from build123d import *

# Parameters (mm, degrees)
SKETCH1_R           = 1
BOSS_EXTRUDE1_DEPTH = 7
SKETCH1_3_R         = 1
BOSS_EXTRUDE2_DEPTH = 2
CUT_EXTRUDE1_DEPTH  = 9
CUT_EXTRUDE2_DEPTH  = 9
FILLET1_R           = 1
FILLET2_R           = 0.3


with BuildPart() as part:
    # Sketch1 → Boss-Extrude1 (new body)
    with BuildSketch(Plane(origin=(0, 0, 0), x_dir=(1, 0, 0), z_dir=(0, 1, 0))):
        with BuildLine():
            Line((117.612796898, 55.564187288), (111.339376302, 55.564187288))
            ThreePointArc((111.339376302, 55.564187288), (106.112953139, 55.838092519), (100.943791761, 56.656807251))
            Line((100.943791761, 56.656807251), (93.116240963, 58.320604535))
            ThreePointArc((93.116240963, 58.320604535), (92.008917517, 58.523581436), (90.891927529, 58.66393173))
            ThreePointArc((90.891927529, 58.66393173), (85.705266175, 59.223876454), (80.531767276, 59.894624719))
            Line((80.531767276, 59.894624719), (9.710099744, 69.847960989))
            ThreePointArc((9.710099744, 69.847960989), (1.798579876, 67.948573115), (-2.692160046, 61.163805184))
            Line((-2.692160046, 61.163805184), (-12.641867563, 14.354111424))
            ThreePointArc((-12.641867563, 14.354111424), (-11.552749071, 6.774676472), (-5.81501604, 1.703933634))
            Line((-5.81501604, 1.703933634), (96.882509001, -38.318979169))
            ThreePointArc((96.882509001, -38.318979169), (102.430072126, -39.906444336), (108.175414493, -40.4417418))
            Line((108.175414493, -40.4417418), (114.4760866, -40.4417418))
            Line((114.4760866, -40.4417418), (120.776758707, -40.4417418))
            ThreePointArc((120.776758707, -40.4417418), (126.522101074, -39.906444336), (132.069664199, -38.318979169))
            Line((132.069664199, -38.318979169), (234.76718924, 1.703933634))
            ThreePointArc((234.76718924, 1.703933634), (240.504922271, 6.774676472), (241.594040763, 14.354111424))
            Line((241.594040763, 14.354111424), (231.644333246, 61.163805184))
            ThreePointArc((231.644333246, 61.163805184), (227.153593324, 67.948573115), (219.242073456, 69.847960989))
            Line((219.242073456, 69.847960989), (148.420405924, 59.894624719))
            ThreePointArc((148.420405924, 59.894624719), (143.246907025, 59.223876454), (138.060245671, 58.66393173))
            ThreePointArc((138.060245671, 58.66393173), (136.943255683, 58.523581436), (135.835932237, 58.320604535))
            Line((135.835932237, 58.320604535), (128.008381439, 56.656807251))
            ThreePointArc((128.008381439, 56.656807251), (122.839220061, 55.838092519), (117.612796898, 55.564187288))
        make_face()
        with Locations(Location((85.734306388, -31.29120092, 0), (0, 0, 270))):
            Circle(SKETCH1_R, mode=Mode.SUBTRACT)
        with Locations(Location((-4.907226209, 4.033293551, 0), (0, 0, 270))):
            Circle(SKETCH1_R, mode=Mode.SUBTRACT)
        with Locations(Location((-10.19649856, 13.834332199, 0), (0, 0, 270))):
            Circle(SKETCH1_R, mode=Mode.SUBTRACT)
        with BuildLine():
            Line((9.01423424, 64.896620645), (79.835901771, 54.943284375))
            ThreePointArc((79.835901771, 54.943284375), (93.947589546, 53.369014537), (108.1260866, 52.602021276))
            Line((108.1260866, 52.602021276), (120.8260866, 52.602021276))
            ThreePointArc((120.8260866, 52.602021276), (135.004583654, 53.369014537), (149.116271429, 54.943284375))
            Line((149.116271429, 54.943284375), (219.93793896, 64.896620645))
            ThreePointArc((219.93793896, 64.896620645), (224.28571114, 63.852812894), (226.753595242, 60.124246735))
            Line((226.753595242, 60.124246735), (236.703302758, 13.314552975))
            ThreePointArc((236.703302758, 13.314552975), (236.104778182, 9.149277911), (232.951609579, 6.362653468))
            Line((232.951609579, 6.362653468), (130.254084538, -33.660259335))
            Line((130.254084538, -33.660259335), (123.992602822, -36.100461634))
            ThreePointArc((123.992602822, -36.100461634), (123.100711644, -36.355681114), (122.177023161, -36.4417418))
            Line((122.177023161, -36.4417418), (120.9760866, -36.4417418))
            Line((120.9760866, -36.4417418), (119.4760866, -36.4417418))
            Line((119.4760866, -36.4417418), (114.4760866, -36.4417418))
            Line((114.4760866, -36.4417418), (109.4760866, -36.4417418))
            Line((109.4760866, -36.4417418), (107.9760866, -36.4417418))
            Line((107.9760866, -36.4417418), (106.775150039, -36.4417418))
            ThreePointArc((106.775150039, -36.4417418), (105.851461556, -36.355681114), (104.959570378, -36.100461634))
            Line((104.959570378, -36.100461634), (98.698088662, -33.660259335))
            Line((98.698088662, -33.660259335), (-3.999436379, 6.362653468))
            ThreePointArc((-3.999436379, 6.362653468), (-7.152604982, 9.149277911), (-7.751129558, 13.314552975))
            Line((-7.751129558, 13.314552975), (2.198577958, 60.124246735))
            ThreePointArc((2.198577958, 60.124246735), (4.66646206, 63.852812894), (9.01423424, 64.896620645))
        make_face(mode=Mode.SUBTRACT)
        with Locations(Location((143.217866812, -31.29120092, 0), (0, 0, 270))):
            Circle(SKETCH1_R, mode=Mode.SUBTRACT)
        with Locations(Location((233.859399409, 4.033293551, 0), (0, 0, 270))):
            Circle(SKETCH1_R, mode=Mode.SUBTRACT)
        with Locations(Location((239.14867176, 13.834332199, 0), (0, 0, 270))):
            Circle(SKETCH1_R, mode=Mode.SUBTRACT)
        with Locations(Location((-0.246791044, 60.64402596, 0), (0, 0, 270))):
            Circle(SKETCH1_R, mode=Mode.SUBTRACT)
        with Locations(Location((9.362166992, 67.372290817, 0), (0, 0, 270))):
            Circle(SKETCH1_R, mode=Mode.SUBTRACT)
        with Locations(Location((90.650187482, 56.175646828, 0), (0, 0, 270))):
            Circle(SKETCH1_R, mode=Mode.SUBTRACT)
        with Locations(Location((138.301985718, 56.175646828, 0), (0, 0, 270))):
            Circle(SKETCH1_R, mode=Mode.SUBTRACT)
        with Locations(Location((229.198964244, 60.64402596, 0), (0, 0, 270))):
            Circle(SKETCH1_R, mode=Mode.SUBTRACT)
        with Locations(Location((219.590006208, 67.372290817, 0), (0, 0, 270))):
            Circle(SKETCH1_R, mode=Mode.SUBTRACT)
    extrude(amount=BOSS_EXTRUDE1_DEPTH)

    # Sketch1_3 → Boss-Extrude2 (add)
    with BuildSketch(Plane(origin=(0, 0, 0), x_dir=(1, 0, 0), z_dir=(0, 1, 0))):
        with BuildLine():
            ThreePointArc((108.1260866, 52.602021276), (93.947589546, 53.369014537), (79.835901771, 54.943284375))
            Line((79.835901771, 54.943284375), (9.01423424, 64.896620645))
            ThreePointArc((9.01423424, 64.896620645), (4.66646206, 63.852812894), (2.198577958, 60.124246735))
            Line((2.198577958, 60.124246735), (-7.751129558, 13.314552975))
            ThreePointArc((-7.751129558, 13.314552975), (-7.152604982, 9.149277911), (-3.999436379, 6.362653468))
            Line((-3.999436379, 6.362653468), (104.959570378, -36.100461634))
            ThreePointArc((104.959570378, -36.100461634), (105.851461556, -36.355681114), (106.775150039, -36.4417418))
            Line((106.775150039, -36.4417418), (122.177023161, -36.4417418))
            ThreePointArc((122.177023161, -36.4417418), (123.100711644, -36.355681114), (123.992602822, -36.100461634))
            Line((123.992602822, -36.100461634), (232.951609579, 6.362653468))
            ThreePointArc((232.951609579, 6.362653468), (236.104778182, 9.149277911), (236.703302758, 13.314552975))
            Line((236.703302758, 13.314552975), (226.753595242, 60.124246735))
            ThreePointArc((226.753595242, 60.124246735), (224.28571114, 63.852812894), (219.93793896, 64.896620645))
            Line((219.93793896, 64.896620645), (149.116271429, 54.943284375))
            ThreePointArc((149.116271429, 54.943284375), (135.004583654, 53.369014537), (120.8260866, 52.602021276))
            Line((120.8260866, 52.602021276), (108.1260866, 52.602021276))
        make_face()
        with Locations(Location((-10.19649856, 13.834332199, 0), (0, 0, 270))):
            Circle(SKETCH1_3_R)
        with Locations(Location((239.14867176, 13.834332199, 0), (0, 0, 270))):
            Circle(SKETCH1_3_R)
        with Locations(Location((-0.246791044, 60.64402596, 0), (0, 0, 270))):
            Circle(SKETCH1_3_R)
        with Locations(Location((229.198964244, 60.64402596, 0), (0, 0, 270))):
            Circle(SKETCH1_3_R)
        with Locations(Location((143.217866812, -31.29120092, 0), (0, 0, 270))):
            Circle(SKETCH1_3_R)
        with Locations(Location((85.734306388, -31.29120092, 0), (0, 0, 270))):
            Circle(SKETCH1_3_R)
        with Locations(Location((9.362166992, 67.372290817, 0), (0, 0, 270))):
            Circle(SKETCH1_3_R)
        with Locations(Location((90.650187482, 56.175646828, 0), (0, 0, 270))):
            Circle(SKETCH1_3_R)
        with Locations(Location((138.301985718, 56.175646828, 0), (0, 0, 270))):
            Circle(SKETCH1_3_R)
        with Locations(Location((219.590006208, 67.372290817, 0), (0, 0, 270))):
            Circle(SKETCH1_3_R)
        with Locations(Location((-4.907226209, 4.033293551, 0), (0, 0, 270))):
            Circle(SKETCH1_3_R)
        with Locations(Location((233.859399409, 4.033293551, 0), (0, 0, 270))):
            Circle(SKETCH1_3_R)
    extrude(amount=BOSS_EXTRUDE2_DEPTH)

    # Sketch2 → Cut-Extrude1 (cut)
    with BuildSketch(Plane(origin=(0, 0, -55.564187288), x_dir=(-1, 0, 0), z_dir=(0, 0, -1))):
        Polygon((-114.4760866, 7), (-120.4760866, 7), (-120.4760866, 3.5), (-114.4760866, 3.5), (-108.4760866, 3.5), (-108.4760866, 7), align=None)
    extrude(amount=-CUT_EXTRUDE1_DEPTH, mode=Mode.SUBTRACT)

    # Sketch2_2 → Cut-Extrude2 (cut)
    with BuildSketch(Plane(origin=(0, 0, -55.564187288), x_dir=(-1, 0, 0), z_dir=(0, 0, -1))):
        Polygon((-114.4760866, 7), (-120.4760866, 7), (-120.4760866, 3.5), (-114.4760866, 3.5), (-108.4760866, 3.5), (-108.4760866, 7), align=None)
    extrude(amount=CUT_EXTRUDE2_DEPTH, mode=Mode.SUBTRACT)

    # Fillet1
    fillet1_edges = [part.edges().sort_by_distance(p)[0] for p in [
        (114.4760866, 3.5, -55.564187288),
        (119.045029455, 3.5, -55.584704398),
        (120.4760866, 5.25, -55.646238892),
        (109.907143745, 3.5, -55.584704398),
        (108.4760866, 5.25, -55.646238892),
    ]]
    fillet(fillet1_edges, radius=FILLET1_R)

    # Fillet2
    fillet2_edges = [part.edges().sort_by_distance(p)[0] for p in [
        (85.705266175, 7, -59.223876454),
        (45.12093351, 7, -64.871292854),
        (1.798579876, 7, -67.948573115),
        (-7.667013804, 7, -37.758958304),
        (-11.552749071, 7, -6.774676472),
        (45.533746481, 7, 18.307522768),
        (102.430072126, 7, 39.906444336),
        (114.4760866, 7, 40.4417418),
        (126.522101074, 7, 39.906444336),
        (183.418426719, 7, 18.307522768),
        (240.504922271, 7, -6.774676472),
        (236.619187004, 7, -37.758958304),
        (227.153593324, 7, -67.948573115),
        (183.83123969, 7, -64.871292854),
        (143.246907025, 7, -59.223876454),
        (136.943255683, 7, -58.523581436),
        (131.922156838, 7, -57.488705893),
        (120.4760866, 7, -53.656371339),
        (108.4760866, 7, -53.656371339),
        (124.720214054, 7, -56.071918989),
        (120.742686716, 7, -55.390518879),
        (108.209486484, 7, -55.390518879),
        (104.231959146, 7, -56.071918989),
        (97.030016362, 7, -57.488705893),
        (92.008917517, 7, -58.523581436),
    ]]
    fillet(fillet2_edges, radius=FILLET2_R)


solid = part.part
CAD build for the part. Positions are in the model's coordinates, mm. A direction names the side the tool comes from. Coordinates: 2 decimals unless noted, no trailing zeros. Answer in a Markdown table with one row per item.
1) Mould opens along Z. For faces 4 (the face through (85.778, 3.303, -59.215)), 5 (the face through (126, 3, 40)), 6 (the face through (4.614, 4.465, -63.816)) say: pulls with the +Z half, pulls with the -Z half, needs draft (parallel to the pull), parting line crosses it, or undercut.
Check values:
| item | result |
|---|---|
| face 4 | pulls with the -Z half |
| face 5 | pulls with the +Z half |
| face 6 | undercut |
2) Which spindle directions (+Z, -Z, +X, -X, +Y, -Y) get a long thin tool onto all of the face, cutting with end or side? Do faces 1 (the face through (224.23, 4.46, -63.89)), 2 (the face through (45.62, 3.3, -64.8)), 3 (the face through (44.613, 6.914, -64.852)). Say none if no direction does.
Check values:
| item | result |
|---|---|
| face 1 | +Y |
| face 2 | -Z, +Y, -Y |
| face 3 | -Z, +Y |
3) Flat gauge pins, fed straight in: P1, Ø1.5, axis at x = 71.5, y = 5.5, coming from the -Z side; P2, Ø1.8, axis at x = 143.22, z = 31.29, coming from the +Y side; P3, Ø3, axis at x = 186, y = 3.5, coming from the +Z side. Where does each tip first touch, or does it go through?
Check values:
| item | result |
|---|---|
| P1 | z = -61.27 |
| P2 | y = 2 |
| P3 | z = 17.89 |
4) Band-saw the part on A-A (y = 5.5). Give the number of separate pieces and of enclosed holes in the cut face, and give its area (3 significant figures).
Check values:
| item | result |
|---|---|
| separate pieces | 1 |
| enclosed holes | 12 |
| area | 2,900 mm2 |
5) Drill centre lines: line 1 (Z direction, x = 8.5, y = 2.75); line 2 (Z direction, x = 72.5, y = 2.25); line 3 (Y direction, x = 112, z = -29.5). Where is each one in solid material? Low to high.
Check values:
| item | result |
|---|---|
| line 1 | -69.95 to -67.88, -66.87 to -64.95, -1.49 to 3.87 |
| line 2 | -61.02 to -55.97, 23.45 to 28.82 |
| line 3 | 0 to 2 |
